Autodesk Inventor part; units mm, degrees
ref_plane "YZ Plane" through (0, 0, 0) normal (1, 0, 0) x (0, 1, 0)
ref_plane "XZ Plane" through (0, 0, 0) normal (0, 1, 0) x (-1, 0, 0)
ref_plane "XY Plane" through (0, 0, 0) normal (0, 0, 1) x (1, 0, 0)
sketch "Sketch1" plane through (0, 0, 0) normal (0, 1, 0) x (-1, 0, 0)
  circle A0 centre (0, 0) radius 25.4
  dimension "d0" = 50.8
extrude "Extrusion1" add sketch "Sketch1" along normal blind 2.8575
fillet "Fillet1" radius 0.635 1 edges at (25.4, 2.8575, 0)
fillet "Fillet2" radius 0.635 1 edges at (25.4, 0, 0)
sketch "Sketch2" plane through (0, 2.8575, 0) normal (0, 1, 0) x (1, 0, 0)
  circle A0 centre (0, 0) radius 24.765
  circle A1 centre (0, 0) radius 6.35
  circle A2 centre (0, 0) radius 15.24
  dimension "d5" = 12.7
  dimension "d6" = 30.48
extrude "Extrusion2" add sketch "Sketch2" along normal blind 128.5875 contours A2
fillet "Fillet3" radius 0.635 1 edges at (-15.24, 131.445, 0)
sketch "Sketch5" plane through (0, 0, 0) normal (0, -1, 0) x (1, 0, 0)
  circle A0 centre (0, 0) radius 24.765
  circle A1 centre (0, 0) radius 6.35
  dimension "d34" = 12.7
extrude "Extrusion4" cut sketch "Sketch5" against normal blind 1.27 contours A1
properties part number "GripFinal" material "Rubber"
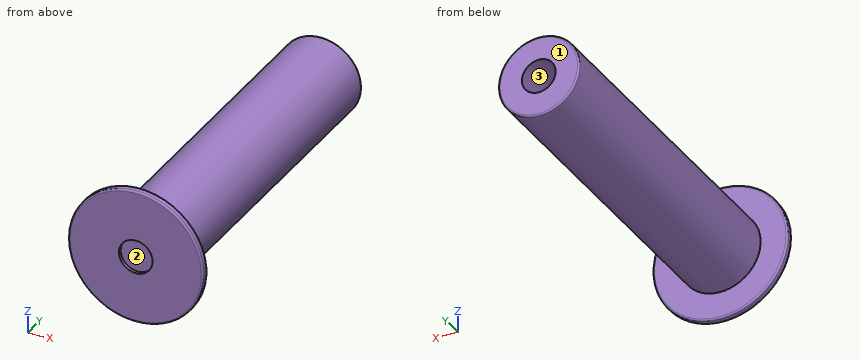
Design review of the part built by this model. Coordinates are the model's own, in mm. Face numbers are marked on the shaded views. A direction names the side the tool comes from. Give positions to 0.01 mm unless a question says otherwise; leave off trailing zeros. Write each loop counter-clockwise with the first axis right and the second up, starting at its lowest first coordinate (ties: lowest second). Pieces come first, ordered by that corner, then holes. Notation, with made-up numbers: M 80.25,70.25 L 110.25,70.25 A19 cw 110.25,92.25 Z; hole C -14.5,35 d10. An arc over 180 degrees is marked long. Return JSON: item names as keys, results as strings. Group by question number.
Item 1: Clearance check with flat-ended pins moving along their axes: pin 1 Ø12 at (x, y) = (-14.5, 54.5) entering from -Z; pin 2 Ø1.5 at (x, y) = (-14.5, 104) entering from -Z; pin 3 Ø8 at (y, z) = (104, 4) entering from -X. State where each tip first meets the part, or that it passes through.
Item 2: Take a section at B-B (y = 102.5). Give the boundary of the cut face in (x, z), plus the area to 3 significant figures.
Item 3: Wall thickness on line 1 along Z through (x, y) = (0, 0.8); line 2 along X through (y, z) = (70, 0); line 3 along Y through (x, z) = (-11.5, 15): over which ranges is each line inside the solid? List them lowest first.
Item 4: Tool access review of the marked faces 1, 2 and 3: name each direction out of +Z, -Z, +X, -X, +Y, -Y from which nothing blocks a thin tool from reaching the whole face with its end or side.
Return value:
{
 "1": {"pin 1": "stops at z = -12.65", "pin 2": "stops at z = -6.57", "pin 3": "stops at x = -15.24"},
 "2": {"outline": "C 0,0 d30.48; hole C 0,0 d12.7", "area": "603 mm2"},
 "3": {"line 1": "z = -25.4 to -6.35, 6.35 to 25.4", "line 2": "x = -15.24 to -6.35, 6.35 to 15.24", "line 3": "y = 0 to 2.86"},
 "4": {"face 1": "+Z, -Z, +X, -X, +Y", "face 2": "-Y", "face 3": "+Y"}
}
